```python
from build123d import *

# Parameters (mm, degrees)
SCHIZZO2_R                   = 3.5
ESTRUSIONE_ESTRUSIONE1_DEPTH = 8


with BuildPart() as part:
    # Schizzo2 → Estrusione-Estrusione1 (new body)
    with BuildSketch(Plane(origin=(0, 0, 0), x_dir=(0, 0, -1), z_dir=(1, 0, 0))):
        with BuildLine():
            Line((17.443402623, -4.562120686), (18.692856186, -4.888900849))
            ThreePointArc((18.692856186, -4.888900849), (24.793396334, -7.641998704), (29.6440016, -12.25369757))
            Line((29.6440016, -12.25369757), (46.600035601, -34.907756452))
            ThreePointArc((46.600035601, -34.907756452), (60.913978484, -42.85118293), (76.365363597, -37.443624966))
            Line((76.365363597, -37.443624966), (82.753482475, -31.392779069))
            ThreePointArc((82.753482475, -31.392779069), (91.534986316, -26.540938387), (101.567665057, -26.563850861))
            Line((101.567665057, -26.563850861), (114.943402623, -30.062120686))
            ThreePointArc((114.943402623, -30.062120686), (122.105106749, -37.2738887), (119.255032306, -47.029742304))
            Line((119.255032306, -47.029742304), (49.969227683, -112.029742304))
            ThreePointArc((49.969227683, -112.029742304), (40.580232317, -114.406888859), (33.580509124, -107.713015918))
            Line((33.580509124, -107.713015918), (5.366313747, -17.213015918))
            ThreePointArc((5.366313747, -17.213015918), (7.679922234, -7.331584183), (17.443402623, -4.562120686))
        make_face()
        with Locations((14.913125179, -14.236710913)):
            Circle(SCHIZZO2_R, mode=Mode.SUBTRACT)
        with Locations((112.413125179, -39.736710913)):
            Circle(SCHIZZO2_R, mode=Mode.SUBTRACT)
        with Locations((43.127320556, -104.736710913)):
            Circle(SCHIZZO2_R, mode=Mode.SUBTRACT)
    extrude(amount=ESTRUSIONE_ESTRUSIONE1_DEPTH)


solid = part.part
```
Source: CAD feature listing. Evaluate the final solid. Frame: model axes, mm. A direction names the side the tool comes from. Give positions to 0.01 mm unless a question says otherwise; leave off trailing zeros. Loops run counter-clockwise (first coordinate to the right, second up) from the corner with the lowest first, then second, coordinate; pieces in that order, holes last. Notation, with made-up numbers: (-38.5, 25.25) -> (-10.5, 25.25) arc R5 cw to (-10.5, 34.25) -> close; hole circle Ø5 at (24.5, 68.25). An arc over 180 degrees is marked (long way). Use a Markdown table: item, result. Add a question column.
(1) Section query D-D (z = -68.5). Output: boundary loops of the cut face in (x, y), then the cut area to 3 significant figures.
(2) Pull-direction query (Y, two-part tool) for faces 1 (the face through (4, -34, -80)), 2 (the face through (3.944, -15.577, -18.146)), 3 (the face through (8, -59, -51)); classes: +Y half, -Y half, draft (parallel to the pull), parting line (faces both ways), or undercut.
(3) Access query for faces 4 (the face through (3.94, -23.42, -38)), 5 (the face through (3.944, -114.442, -40.717)). Directions: +Z, -Z, +X, -X, +Y, -Y. A direction counts if a zero-diameter tool reaches every point of the face in a straight line with its end or side. Return the directions, or none.
(4) Ray query, line 1 (Y direction, x = 0.75, z = -44); line 2 (Y direction, x = 5, z = -114.5); line 3 (Z direction, x = 6.75, y = -106). Return the intervals inside material, ascending.
(5) Section query A-A (z = -14.5). Output: boundary loops of the cut face in (x, y), then the cut area to 3 significant figures.
(6) Section query B-B (x = 6). Output: boundary loops of the cut face in (y, z).
(7) Section query C-C (y = -67). Output: boundary loops of the cut face in (x, z).
(8) First-contact query: pin 1 Ø4 at (y, z) = (-94, -75) entering from -X. Flat tip, straight axial feed; report the tip coordinate or a pass-through.
Checked values:
| question | item | result |
|---|---|---|
| 1 | outline | (0, -94.65) -> (8, -94.65) -> (8, -42.04) -> (0, -42.04) -> close |
| 1 | area | 421 mm^2 |
| 2 | face 1 | +Y half |
| 2 | face 2 | undercut |
| 2 | face 3 | draft |
| 3 | face 4 | +X, -X, +Y |
| 3 | face 5 | +X, -X, -Y |
| 4 | line 1 | -114.7 to -108.13, -101.35 to -31.43 |
| 4 | line 2 | -51.49 to -42.55, -36.93 to -29.95 |
| 4 | line 3 | -56.4 to -46.39, -39.86 to -33.05 |
| 5 | outline | (0, -46.51) -> (8, -46.51) -> (8, -17.71) -> (0, -17.71) -> close; (0, -10.76) -> (8, -10.76) -> (8, -4.25) -> (0, -4.25) -> close |
| 5 | area | 283 mm^2 |
| 6 | outline | (-112.03, -49.97) -> (-47.03, -119.26) arc R10 ccw to (-30.06, -114.94) -> (-26.56, -101.57) arc R20 ccw to (-31.39, -82.75) -> (-37.44, -76.37) arc R20 cw to (-34.91, -46.6) -> (-12.25, -29.64) arc R20 ccw to (-4.89, -18.69) -> (-4.56, -17.44) arc R10 ccw to (-17.21, -5.37) -> (-107.71, -33.58) arc R10 ccw to start; hole circle Ø7 at (-104.74, -43.13); hole circle Ø7 at (-39.74, -112.41); hole circle Ø7 at (-14.24, -14.91) |
| 7 | outline | (0, -97.97) -> (8, -97.97) -> (8, -20.89) -> (0, -20.89) -> close |
| 8 | pin 1 | through |
